from build123d import *

# Parameters (mm, degrees)
SKETCH1_R           = 3.1
BOSS_EXTRUDE1_DEPTH = 3
CUT_EXTRUDE1_DEPTH  = 335.294780097
FILLET1_R           = 45
SKETCH3_R           = 10
CUT_EXTRUDE2_DEPTH  = 335.294780097
SKETCH4_R           = 2.6
CUT_EXTRUDE3_DEPTH  = 335.294780097
SKETCH5_R           = 1.6
CUT_EXTRUDE4_DEPTH  = 335.294780097
SKETCH6_R           = 1.6
CUT_EXTRUDE5_DEPTH  = 335.294780097


with BuildPart() as part:
    # Sketch1 → Boss-Extrude1 (new body)
    # profile 1 of 2: a face of its own
    with BuildSketch(Plane(origin=(0, 0, 0), x_dir=(1, 0, 0), z_dir=(0, 1, 0))):
        with BuildLine():
            Line((0, -52), (260, -52))
            ThreePointArc((260, -52), (312, 0), (260, 52))
            Line((260, 52), (0, 52))
            ThreePointArc((0, 52), (-52, 0), (0, -52))
        make_face()
        with Locations(Location((0, 0, 0), (0, 0, 270))):
            Circle(SKETCH1_R, mode=Mode.SUBTRACT)
        with BuildLine():
            ThreePointArc((250, 3.1), (246.9, 0), (250, -3.1))
            Line((250, -3.1), (270, -3.1))
            ThreePointArc((270, -3.1), (273.1, 0), (270, 3.1))
            Line((270, 3.1), (250, 3.1))
        make_face(mode=Mode.SUBTRACT)
    # profile 2 of 2: a face of its own
    with BuildSketch(Plane(origin=(0, 0, 0), x_dir=(1, 0, 0), z_dir=(0, 1, 0))):
        with BuildLine():
            ThreePointArc((-52, 0), (-36.769552622, 36.769552622), (0, 52))
            Line((0, 52), (260, 52))
            ThreePointArc((260, 52), (296.769552622, 36.769552622), (312, 0))
            Line((312, 0), (312, 120))
            Line((312, 120), (-52, 120))
            Line((-52, 120), (-52, 0))
        make_face()
    extrude(amount=BOSS_EXTRUDE1_DEPTH)

    # Sketch2 → Cut-Extrude1 (cut, through all)
    with BuildSketch(Plane(origin=(0, 3, 0), x_dir=(1, 0, 0), z_dir=(0, 1, 0))):
        with BuildLine():
            Line((87.4, -37), (87.4, 98))
            ThreePointArc((87.4, 98), (90, 100.6), (92.6, 98))
            Line((92.6, 98), (92.6, -37))
            ThreePointArc((92.6, -37), (90, -39.6), (87.4, -37))
        make_face()
        with BuildLine():
            Line((172.6, -37), (172.6, 98))
            ThreePointArc((172.6, 98), (170, 100.6), (167.4, 98))
            Line((167.4, 98), (167.4, -37))
            ThreePointArc((167.4, -37), (170, -39.6), (172.6, -37))
        make_face()
    extrude(amount=-CUT_EXTRUDE1_DEPTH, mode=Mode.SUBTRACT)

    # Fillet1
    fillet1_edges = [part.edges().sort_by_distance(p)[0] for p in [
        (-52, 1.5, -120),
        (312, 1.5, -120),
    ]]
    fillet(fillet1_edges, radius=FILLET1_R)

    # Sketch3 → Cut-Extrude2 (cut, through all)
    with BuildSketch(Plane(origin=(0, 3, 0), x_dir=(1, 0, 0), z_dir=(0, 1, 0))):
        with Locations(Location((0, 0, 0), (0, 0, 270))):
            Circle(SKETCH3_R)
    extrude(amount=-CUT_EXTRUDE2_DEPTH, mode=Mode.SUBTRACT)

    # Sketch4 → Cut-Extrude3 (cut, through all)
    with BuildSketch(Plane.XZ):
        with Locations(Location((17.4, -100.4, 0), (0, 0, 270))):
            Circle(SKETCH4_R)
        with Locations(Location((27.4, -100.4, 0), (0, 0, 270))):
            Circle(SKETCH4_R)
        with Locations(Location((232.4, -100.4, 0), (0, 0, 270))):
            Circle(SKETCH4_R)
        with Locations(Location((242.4, -100.4, 0), (0, 0, 270))):
            Circle(SKETCH4_R)
    extrude(amount=-CUT_EXTRUDE3_DEPTH, mode=Mode.SUBTRACT)

    # Sketch5 → Cut-Extrude4 (cut, through all)
    with BuildSketch(Plane(origin=(0, 3, 0), x_dir=(1, 0, 0), z_dir=(0, 1, 0))):
        with Locations(Location((-17.5, 0, 0), (0, 0, 270))):
            Circle(SKETCH5_R)
        with Locations(Location((17.5, 0, 0), (0, 0, 270))):
            Circle(SKETCH5_R)
    extrude(amount=-CUT_EXTRUDE4_DEPTH, mode=Mode.SUBTRACT)

    # Sketch6 → Cut-Extrude5 (cut, through all)
    with BuildSketch(Plane(origin=(0, 3, 0), x_dir=(1, 0, 0), z_dir=(0, 1, 0))):
        with Locations(Location((-13.5, -35, 0), (0, 0, 270))):
            Circle(SKETCH6_R)
        with Locations(Location((4.5, -35, 0), (0, 0, 270))):
            Circle(SKETCH6_R)
        with Locations(Location((255.5, -35, 0), (0, 0, 270))):
            Circle(SKETCH6_R)
        with Locations(Location((273.5, -35, 0), (0, 0, 270))):
            Circle(SKETCH6_R)
    extrude(amount=-CUT_EXTRUDE5_DEPTH, mode=Mode.SUBTRACT)


solid = part.part
Verification items for the finished model (mm, model axes). Give positions to 0.01 mm unless a question says otherwise; leave off trailing zeros. Order: outer loops, then holes, each group sorted by start corner. A loop starts at its lowest first (then second) coordinate and runs counter-clockwise, first axis right, second up. Notation, with made-up numbers: M 12.25,-6 L 50.25,-6 A22 ccw 50.25,10 Z; hole C -8.75,8 d8. An arc over 180 degrees is marked long. Answer as a JSON object with one key per item and string values. Group by question number.
1) Cross-section at C-C (z = -79). Enter the section's corners in (x, y).
2) Mould release check, pull along X, two halves, no side actions. Record for faces 1 (the face through (127, 0, -35)), 2 (the face through (-9.76, 1.52, -2.17)), 3 (the face through (-37.172, 1.479, 36.363)), 4 (the face through (296.363, 1.479, 37.172)): released by +X, released by -X, zero draft, split by the parting line, or undercut.
3) Scan lines: line 1 along Z through (x, y) = (255.5, 1.75); line 2 along X through (y, z) = (0.85, -13.5); line 3 along X through (y, z) = (0.7, 10.5). Record each from-to range of solid material in increasing order. Write a range as [from, to].
4) Cross-section at A-A (z = -42). Enter the section's corners in (x, y), then the cut area to 3 significant figures.
5) Cross-section at B-B (y = 2.3). Give the number of separate pieces and of enclosed holes in the cut face, then the cut area to 3 significant figures.
6) Depth check by flat-ended pin: pin 1 Ø4.5 at (x, z) = (27.4, -100.4) entering from -Y. Enter the tip coordinate at first touch or a pass-through.
Result sheet:
{
 "1": {"outline": "M -51.82,0 L 87.4,0 L 87.4,3 L -51.82,3 Z; M 92.6,0 L 167.4,0 L 167.4,3 L 92.6,3 Z; M 172.6,0 L 311.82,0 L 311.82,3 L 172.6,3 Z"},
 "2": {"face 1": "zero draft", "face 2": "undercut", "face 3": "released by -X", "face 4": "released by +X"},
 "3": {"line 1": "z = [-120, -3.1], [3.1, 33.4], [36.6, 52]", "line 2": "x = [-52, 87.4], [92.6, 167.4], [172.6, 312]", "line 3": "x = [-50.93, 87.4], [92.6, 167.4], [172.6, 310.93]"},
 "4": {"outline": "M -52,0 L 87.4,0 L 87.4,3 L -52,3 Z; M 92.6,0 L 167.4,0 L 167.4,3 L 92.6,3 Z; M 172.6,0 L 312,0 L 312,3 L 172.6,3 Z", "area": "1,060 mm2"},
 "5": {"separate pieces": "1", "enclosed holes": "14", "area": "58,500 mm2"},
 "6": {"pin 1": "passes through"}
}
